```python
from build123d import *

# Parameters (mm, degrees)
ESQUISSE1_R                                        = 1.2
ESQUISSE1_R_2                                      = 11.5
ESQUISSE1_R_3                                      = 1
BOSS_EXTRU_1_DEPTH                                 = 4
CHAMBRAGE_POUR_VIS_T_TE_RONDE_BOMB_E_M_D           = 2.9
CHAMBRAGE_POUR_VIS_T_TE_RONDE_BOMB_E_M_CBORE_D     = 6
CHAMBRAGE_POUR_VIS_T_TE_RONDE_BOMB_E_M_CBORE_DEPTH = 2.1
CONG_1_R                                           = 1
D_GAGEMENT_M34_D                                   = 3.4
CHAMBRAGE_POUR_VIS_T_TE_RONDE_BOMB_2_D             = 2.9
CHAMBRAGE_POUR_VIS_T_TE_RONDE_BOMB_2_CBORE_D       = 6
CHAMBRAGE_POUR_VIS_T_TE_RONDE_BOMB_2_CBORE_DEPTH   = 2.1
CHAMBRAGE_POUR_VIS_T_TE_RONDE_BOMB_3_D             = 3.4
CHAMBRAGE_POUR_VIS_T_TE_RONDE_BOMB_3_CBORE_D       = 7
CHAMBRAGE_POUR_VIS_T_TE_RONDE_BOMB_3_CBORE_DEPTH   = 2.4


with BuildPart() as part:
    # Esquisse1 → Boss.-Extru.1 (new body)
    with BuildSketch(Plane.XY):
        with BuildLine():
            Line((55.801816314, -15.329976162), (-55.801816314, -15.329976162))
            Line((-55.801816314, -15.329976162), (-55.801816314, 1.670023838))
            ThreePointArc((-55.801816314, 1.670023838), (-41.441556985, 18.934224014), (-32.822029076, 39.670023838))
            Line((-32.822029076, 39.670023838), (32.822029076, 39.670023838))
            ThreePointArc((32.822029076, 39.670023838), (41.441556985, 18.934224014), (55.801816314, 1.670023838))
            Line((55.801816314, 1.670023838), (55.801816314, -15.329976162))
        make_face()
        with Locations((15, -5.410480756)):
            Circle(ESQUISSE1_R, mode=Mode.SUBTRACT)
        with Locations((15, 28.589519244)):
            Circle(ESQUISSE1_R, mode=Mode.SUBTRACT)
        with Locations(Location((-15, -5.410480756, 0), (0, 0, 180))):
            Circle(ESQUISSE1_R, mode=Mode.SUBTRACT)
        with Locations(Location((-15, 28.589519244, 0), (0, 0, 180))):
            Circle(ESQUISSE1_R, mode=Mode.SUBTRACT)
        with Locations((0, -0.910480756)):
            Circle(ESQUISSE1_R_2, mode=Mode.SUBTRACT)
        with Locations((45, -0.910480756)):
            Circle(ESQUISSE1_R_3, mode=Mode.SUBTRACT)
        with Locations((-45, -0.910480756)):
            Circle(ESQUISSE1_R_3, mode=Mode.SUBTRACT)
        with Locations((-8.5, 34.889519244)):
            Circle(ESQUISSE1_R_3, mode=Mode.SUBTRACT)
        with Locations((8.5, 34.889519244)):
            Circle(ESQUISSE1_R_3, mode=Mode.SUBTRACT)
    extrude(amount=BOSS_EXTRU_1_DEPTH)

    # Chambrage pour vis _ t_te ronde bomb_e M (through all)
    with Locations(Plane.XY.offset(4)):
        with Locations((-15, 28.589519244), (15, 28.589519244), (15, -5.410480756), (-15, -5.410480756)):
            CounterBoreHole(CHAMBRAGE_POUR_VIS_T_TE_RONDE_BOMB_E_M_D / 2, CHAMBRAGE_POUR_VIS_T_TE_RONDE_BOMB_E_M_CBORE_D / 2, CHAMBRAGE_POUR_VIS_T_TE_RONDE_BOMB_E_M_CBORE_DEPTH)

    # Congé1
    cong_1_edges = [part.edges().sort_by_distance(p)[0] for p in [
        (-32.822029076, 39.670023838, 2),
        (32.822029076, 39.670023838, 2),
        (55.801816314, 1.670023838, 2),
        (55.801816314, -15.329976162, 2),
        (-55.801816314, -15.329976162, 2),
        (-55.801816314, 1.670023838, 2),
        (0, -15.329976162, 4),
        (55.801816314, -6.829976162, 4),
        (41.441556985, 18.934224014, 4),
        (0, 39.670023838, 4),
        (-41.441556985, 18.934224014, 4),
        (0, 39.670023838, 0),
        (41.441556985, 18.934224014, 0),
        (55.801816314, -6.829976162, 0),
        (0, -15.329976162, 0),
        (-55.801816314, -6.829976162, 0),
        (-41.441556985, 18.934224014, 0),
        (-55.801816314, -6.829976162, 4),
    ]]
    fillet(cong_1_edges, radius=CONG_1_R)

    # Dégagement M34 (through all)
    with Locations(Plane.XY.offset(4)):
        with Locations((-45, -0.910480756), (45, -0.910480756)):
            Hole(D_GAGEMENT_M34_D / 2)

    # Chambrage pour vis _ t_te ronde bomb 2 (through all)
    with Locations(Plane.XY.offset(4)):
        with Locations((-8.5, 34.889519244), (8.5, 34.889519244)):
            CounterBoreHole(CHAMBRAGE_POUR_VIS_T_TE_RONDE_BOMB_2_D / 2, CHAMBRAGE_POUR_VIS_T_TE_RONDE_BOMB_2_CBORE_D / 2, CHAMBRAGE_POUR_VIS_T_TE_RONDE_BOMB_2_CBORE_DEPTH)

    # Chambrage pour vis _ t_te ronde bomb 3 (through all)
    with Locations(Plane(origin=(0, 0, 0), x_dir=(-1, 0, 0), z_dir=(0, 0, -1))):
        with Locations((45, -0.910480756), (-45, -0.910480756)):
            CounterBoreHole(CHAMBRAGE_POUR_VIS_T_TE_RONDE_BOMB_3_D / 2, CHAMBRAGE_POUR_VIS_T_TE_RONDE_BOMB_3_CBORE_D / 2, CHAMBRAGE_POUR_VIS_T_TE_RONDE_BOMB_3_CBORE_DEPTH)


solid = part.part
```
Work out the finished part from the listing and answer in its coordinate system (mm). A direction names the side the tool comes from. Give positions to 0.01 mm unless a question says otherwise; leave off trailing zeros. Loops run counter-clockwise (first coordinate to the right, second up) from the corner with the lowest first, then second, coordinate; pieces in that order, holes last. Notation, with made-up numbers: (7, 24.5) - (58, 24.5) arc R20 cw to (58, 38.5) - close; hole circle Ø6 at (-24.5, 4). An arc over 180 degrees is marked (long way). Use CSV: the item, a comma, the result in double quotes. Start each with the question number.
(1) Determine the mould class of faces 4 (the face through (41.368, 19.057, 1.986)), 5 (the face through (-16, -7, 1.9)), 6 (the face through (1, 13, 0)) for opening direction Y: released by +Y, released by -Y, zero draft, split by the parting line, or undercut.
(2) Each of these flat-tipped pins is pushed along its axis until it touches: pin 1 (12 mm diameter, centred on x = -35, y = -6.5, fed in from -Z); pin 2 (4.5 mm diameter, centred on x = -15, y = -5.41, fed in from +Z); pin 3 (3 mm diameter, centred on x = -45, y = -0.91, fed in from -Z); pin 4 (5.5 mm diameter, centred on x = 45, y = -0.91, fed in from -Z). Where does it stop, or does it pass through?
(3) Find the intervals of material crossed by L1, parallel to Y at x = -15, z = 2.7; L2, parallel to Y at x = -8, z = 0.7; L3, parallel to Y at x = 0, z = 1.3, in increasing order.
(4) Find section B-B, the plane x = 3. Determine the outline of the cut face in (y, z), plus the area to 3 significant figures.
(5) Find section A-A, the plane x = 15. Determine the outline of the cut face in (y, z), plus the area to 3 significant figures.
(6) A tool of negligible diameter and unlimited length cuts with its end or side. For faces 1 (the face through (9.95, 34.95, 0.94)), 2 (the face through (11.27, 33.74, 2.96)), 3 (the face through (43, 0, 2.4)), from which of +Z, -Z, +X, -X, +Y, -Y can it reach the whole face along a straight path? Write none if from no direction.
Results found:
1,face 4,"released by +Y"
1,face 5,"undercut"
1,face 6,"zero draft"
2,pin 1,"z = 0"
2,pin 2,"z = 1.9"
2,pin 3,"through"
2,pin 4,"z = 2.4"
3,L1,"-15.33 to -8.41, -2.41 to 25.59, 31.59 to 39.67"
3,L2,"-15.28 to -9.17, 7.35 to 33.53, 36.25 to 39.62"
3,L3,"-15.33 to -12.41, 10.59 to 39.67"
4,outline,"(-15.33, 1) arc R1 ccw to (-14.33, 0) - (-12.01, 0) - (-12.01, 4) - (-14.33, 4) arc R1 ccw to (-15.33, 3) - close; (10.19, 0) - (38.67, 0) arc R1 ccw to (39.67, 1) - (39.67, 3) arc R1 ccw to (38.67, 4) - (10.19, 4) - close"
4,area,"130 mm^2"
5,outline,"(-15.33, 1) arc R1 ccw to (-14.33, 0) - (-6.86, 0) - (-6.86, 1.9) - (-8.41, 1.9) - (-8.41, 4) - (-14.33, 4) arc R1 ccw to (-15.33, 3) - close; (-3.96, 0) - (27.14, 0) - (27.14, 1.9) - (25.59, 1.9) - (25.59, 4) - (-2.41, 4) - (-2.41, 1.9) - (-3.96, 1.9) - close; (30.04, 0) - (38.67, 0) arc R1 ccw to (39.67, 1) - (39.67, 3) arc R1 ccw to (38.67, 4) - (31.59, 4) - (31.59, 1.9) - (30.04, 1.9) - close"
5,area,"183 mm^2"
6,face 1,"+Z, -Z"
6,face 2,"+Z"
6,face 3,"-Z"
